Check sheet for the modelled part. Datum: model origin and axes. Units: mm. A direction names the side the tool comes from. Round coordinates to 2 decimals unless told otherwise and drop trailing zeros. Order: outer loops, then holes, each group sorted by start corner. A loop starts at its lowest first (then second) coordinate and runs counter-clockwise, first axis right, second up.
```python
from build123d import *

# Parameters (mm, degrees)
F0_R     = 45
F0_R_2   = 4
F1_DEPTH = 12
F2_R     = 4
F3_DEPTH = 3


with BuildPart() as f1:
    # F0 (on Top) → F1 (new body)
    with BuildSketch(Plane.XY):
        Circle(F0_R)
        Circle(F0_R_2, mode=Mode.SUBTRACT)
    extrude(amount=F1_DEPTH)

    # F2 (on face) → F3 (cut)
    with BuildSketch(Plane.XY.offset(12)):
        Polygon((0.459643, -7.491466), (6.717621, -3.347671), (6.257979, 4.143795), (-0.459643, 7.491466), (-6.717621, 3.347671), (-6.257979, -4.143795), align=None)
        Circle(F2_R, mode=Mode.SUBTRACT)
    extrude(amount=-F3_DEPTH, mode=Mode.SUBTRACT)


solid = f1.part
```
Item 1: Access from +Z, -Z, +X, -X, +Y, -Y to the whole of each face (thin tool, end or side, straight path). Record for faces 4 (the flat face through (3.54, -5.45, 10.52)), 5 (the flat face through (-1, -9, 0)).
Answer:
face 4: +Z
face 5: -Z, +X, -X, +Y, -Y
Item 2: Go/stop test with flat-tipped pins: P1, Ø3, axis at y = 31.5, z = 8.5, coming from the -X side; P2, Ø4, axis at x = -16.5, z = 4.5, coming from the +Y side; P3, Ø6, axis at y = -8.5, z = 8.5, coming from the +X side. Record where each tip stops, or that it passes through.
Answer:
P1: stops at x = -33.54
P2: stops at y = 42.6
P3: stops at x = 44.66
Item 3: Release check for a two-part mould opening along X. For faces 1 (the flat face through (-1, -9, 12)), 2 (the flat face through (-3.54, 5.45, 10.52)), 3 (the cylindrical face through (20.765, -39.923, 5.916)) record: released by +X, released by -X, zero draft, split by the parting line, or undercut.
Answer:
face 1: zero draft
face 2: undercut
face 3: split by the parting line
Item 4: Sectioned sample at A-A (y = 0). Record the cut outline in (x, z).
Answer:
outline: (-45, 0) - (-4, 0) - (-4, 9) - (-6.51, 9) - (-6.51, 12) - (-45, 12) - close; (4, 0) - (45, 0) - (45, 12) - (6.51, 12) - (6.51, 9) - (4, 9) - close
Item 5: Scan lines: line 1 along Y through (x, z) = (0, 6.5); line 2 along Z through (x, y) = (-5.5, -0.5); line 3 along X through (y, z) = (-0.5, 10.5). Record each from-to range of solid material in increasing order.
Answer:
line 1: y = -45 to -4, 4 to 45
line 2: z = 0 to 9
line 3: x = -45 to -6.48, 6.54 to 45
Item 6: Sectioned sample at C-C (x = -15). Record the cut outline in (y, z).
Answer:
outline: (-42.43, 0) - (42.43, 0) - (42.43, 12) - (-42.43, 12) - close
Item 7: Sectioned sample at D-D (y = -15.5). Record the cut outline in (x, z).
Answer:
outline: (-42.25, 0) - (42.25, 0) - (42.25, 12) - (-42.25, 12) - close
Item 8: Sectioned sample at B-B (z = 5.25). Record the cut outline in (x, y).
Answer:
outline: circle Ø90 at (0, 0); hole circle Ø8 at (0, 0)
